from build123d import *

# Parameters (mm, degrees)
F0_W     = 89.5604
F0_H     = 89.5604
F1_DEPTH = 203.2
F3_DEPTH = 101.6
F4_R     = 5.08


with BuildPart() as f1:
    # F0 (on Top) → F1 (new body)
    with BuildSketch(Plane.XY):
        Polygon((0, 50.8), (-50.8, 50.8), (-50.8, 0), (-50.8, -50.8), (0, -50.8), (50.8, -50.8), (50.8, 0), (50.8, 50.8), align=None)
        Rectangle(F0_W, F0_H, mode=Mode.SUBTRACT)
    extrude(amount=F1_DEPTH)

    # F2 (on face) → F3 (cut)
    with BuildSketch(Plane.YZ.offset(50.8)):
        Polygon((-12.7, 203.2), (-50.8, 203.2), (-50.8, 181.202955), align=None)
        Polygon((50.8, 203.2), (12.7, 203.2), (50.8, 181.202955), align=None)
    extrude(amount=-F3_DEPTH, mode=Mode.SUBTRACT)

    # F4
    f4_edges = [f1.edges().sort_by_distance(p)[0] for p in [
        (-50.8, -50.8, 90.601477),
        (50.8, -50.8, 90.601477),
        (50.8, 50.8, 90.601477),
        (-44.7802, 44.7802, 92.339244),
        (-44.7802, -44.7802, 92.339244),
        (-50.8, 50.8, 90.601477),
        (44.7802, -44.7802, 92.339244),
        (44.7802, 44.7802, 92.339244),
    ]]
    fillet(f4_edges, radius=F4_R)


solid = f1.part
Work out the finished part from the listing and answer in its coordinate system (mm). A direction names the side the tool comes from. Give positions to 0.01 mm unless a question says otherwise; leave off trailing zeros. Loops run counter-clockwise (first coordinate to the right, second up) from the corner with the lowest first, then second, coordinate; pieces in that order, holes last. Notation, with made-up numbers: M 73,-35.75 L 90,-35.75 A26 cw 90,-7.75 Z; hole C -33,64 d1. An arc over 180 degrees is marked long. Use CSV: the item, a comma, the result in double quotes.
1) Which of the six approach directions +Z, -Z, +X, -X, +Y, -Y give full straight-line access (tool end or side, diameter ignored) to faces 4 (the cylindrical face through (-49.351, 49.272, 93.357)), 5 (the cylindrical face through (-43.253, 43.332, 95.119))?
Answer:
face 4,"+Z, -Z, -X, +Y"
face 5,"+Z, -Z"
2) Given P1, Ø10, axis at x = 39, y = -6.5, coming from the -Z side, flat-ended and moving along its own axis, determine where the tip first touches the part or whether it passes through.
Answer:
P1,"through"
3) Determine the mould class of faces 1 (the cylindrical face through (-49.351, -49.272, 93.357)), 2 (the cylindrical face through (43.332, 43.253, 95.119)), 3 (the flat face through (-3.526, 45.772, 184.106)) for opening direction X: released by +X, released by -X, zero draft, split by the parting line, or undercut.
Answer:
face 1,"released by -X"
face 2,"undercut"
face 3,"zero draft"
4) Find section A-A on x = 9.5. Write down the section's boundary in (y, z).
Answer:
outline,"M -50.8,0 L -44.78,0 L -44.78,184.68 L -50.8,181.2 Z; M 44.78,0 L 50.8,0 L 50.8,181.2 L 44.78,184.68 Z"
5) Find section B-B on y = 2.5. Write down the section's boundary in (x, z).
Answer:
outline,"M -50.8,0 L -44.78,0 L -44.78,203.2 L -50.8,203.2 Z; M 44.78,0 L 50.8,0 L 50.8,203.2 L 44.78,203.2 Z"
6) Consider L1, parallel to Y at x = -15, z = 108; L2, parallel to Z at x = -22, y = -45.5. Determine where each line is inside the solid, lowest interval first.
Answer:
L1,"-50.8 to -44.78, 44.78 to 50.8"
L2,"0 to 184.26"
7) Find section C-C on z = 79.5. Write down the section's boundary in (x, y).
Answer:
outline,"M -50.8,-45.72 A5.08 ccw -45.72,-50.8 L 45.72,-50.8 A5.08 ccw 50.8,-45.72 L 50.8,45.72 A5.08 ccw 45.72,50.8 L -45.72,50.8 A5.08 ccw -50.8,45.72 Z; hole M -44.78,-39.7 A5.08 ccw -39.7,-44.78 L 39.7,-44.78 A5.08 ccw 44.78,-39.7 L 44.78,39.7 A5.08 ccw 39.7,44.78 L -39.7,44.78 A5.08 ccw -44.78,39.7 Z"
